Can you work these out from the model? Positions are in its coordinate system, mm. Face numbers are marked on the shaded views. A direction names the side the tool comes from. Round coordinates to 2 decimals unless told otherwise and drop trailing zeros. Order: outer loops, then holes, each group sorted by start corner. A loop starts at its lowest first (then second) coordinate and runs counter-clockwise, first axis right, second up. Notation, with made-up numbers: (2, -40) -> (35, -40) arc R16 cw to (35, -30) -> close; hole circle Ø11 at (-24, 12). An arc over 180 degrees is marked (long way). Use a Markdown table: item, result. Add a question column.
Q1. For the marked faces 1 and 2, which set-ups out of +Z, -Z, +X, -X, +Y, -Y let a thin tool reach every point of the face, with its end or its side?
Q2. If we section it at B-B on y = 14.75: List the corners of the cut face in (x, z) for me (3 decimals).
Q3. If we section it at D-D on x = 34: List the corners of the cut face in (y, z) for me (3 decimals), plus the area to 3 significant figures.
Q4. If we section it at C-C on x = 27.1: List the corners of the cut face in (y, z) for me (3 decimals), plus the area to 3 significant figures.
Q5. I'm going to push flat-ended pins straight in: pin 1 Ø1 at (x, y) = (8.5, 16) entering from -Z (3 decimals); pin 2 Ø5.5 at (y, z) = (9, -19) entering from +X (3 decimals). Where does each tip first touch, or does it pass through?
Q6. If we section it at A-A on z = -27.1: List the corners of the cut face in (x, y) for me (3 decimals).
Q7. I need wall thicknesses on line 1 along Y through (x, z) = (1.7, -13.1) (3 decimals); line 2 along X through (y, z) = (17, -16) (3 decimals); line 3 along Z through (x, y) = (24.5, 8) (3 decimals). Which ranges of each line are inside material? Lowest first, please. Write a range as [from, to].
```python
from build123d import *

# Parameters (mm, degrees)
BOSS_EXTRUDE1_DEPTH = 19.05
FILLET1_R           = 3
FILLET2_R           = 1
SKETCH2_R           = 1.6
CUT_EXTRUDE1_DEPTH  = 58.15
SKETCH3_R           = 1.6
CUT_EXTRUDE2_DEPTH  = 58.15


with BuildPart() as part:
    # Sketch1 → Boss-Extrude1 (new body)
    with BuildSketch(Plane(origin=(0, 0, 0), x_dir=(1, 0, 0), z_dir=(0, 1, 0))):
        Polygon((0, 0), (0, 38.1), (3.175, 38.1), (3.175, 3.175), (38.1, 3.175), (38.1, 0), align=None)
    extrude(amount=BOSS_EXTRUDE1_DEPTH)

    # Fillet1
    fillet1_edges = [part.edges().sort_by_distance(p)[0] for p in [
        (3.175, 9.525, -38.1),
        (3.175, 9.525, -3.175),
        (38.1, 9.525, -3.175),
    ]]
    fillet(fillet1_edges, radius=FILLET1_R)

    # Fillet2
    fillet2_edges = [part.edges().sort_by_distance(p)[0] for p in [
        (0, 9.525, 0),
    ]]
    fillet(fillet2_edges, radius=FILLET2_R)

    # Sketch2 → Cut-Extrude1 (cut, through all)
    with BuildSketch(Plane.XY):
        with Locations((13.1, 9.525)):
            Circle(SKETCH2_R)
        with Locations((27.1, 9.525)):
            Circle(SKETCH2_R)
    extrude(amount=-CUT_EXTRUDE1_DEPTH, mode=Mode.SUBTRACT)

    # Sketch3 → Cut-Extrude2 (cut, through all)
    with BuildSketch(Plane.ZY):
        with Locations((-27.1, 9.525)):
            Circle(SKETCH3_R)
        with Locations((-13.1, 9.525)):
            Circle(SKETCH3_R)
    extrude(amount=-CUT_EXTRUDE2_DEPTH, mode=Mode.SUBTRACT)


solid = part.part
```
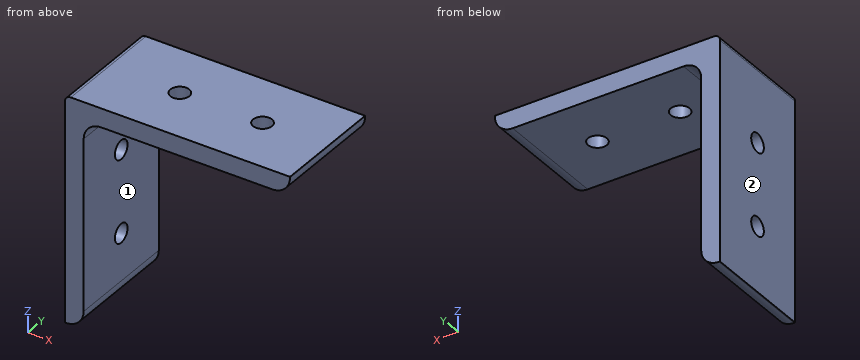
Answer below:
| question | item | result |
|---|---|---|
| 1 | face 1 | -Z, +X, +Y, -Y |
| 1 | face 2 | +Z, -Z, -X, +Y, -Y |
| 2 | outline | (0, -38.1) -> (0.175, -38.1) arc R3 ccw to (3.175, -35.1) -> (3.175, -6.175) arc R3 cw to (6.175, -3.175) -> (35.1, -3.175) arc R3 ccw to (38.1, -0.175) -> (38.1, 0) -> (1, 0) arc R1 ccw to (0, -1) -> close |
| 3 | outline | (0, -3.175) -> (19.05, -3.175) -> (19.05, 0) -> (0, 0) -> close |
| 3 | area | 60.5 mm² |
| 4 | outline | (0, -3.175) -> (7.925, -3.175) -> (7.925, 0) -> (0, 0) -> close; (11.125, -3.175) -> (19.05, -3.175) -> (19.05, 0) -> (11.125, 0) -> close |
| 4 | area | 50.3 mm² |
| 5 | pin 1 | z = -3.175 |
| 5 | pin 2 | x = 3.175 |
| 6 | outline | (0, 0) -> (3.175, 0) -> (3.175, 7.925) -> (0, 7.925) -> close; (0, 11.125) -> (3.175, 11.125) -> (3.175, 19.05) -> (0, 19.05) -> close |
| 7 | line 1 | [0, 7.925], [11.125, 19.05] |
| 7 | line 2 | [0, 3.175] |
| 7 | line 3 | [-3.175, 0] |
